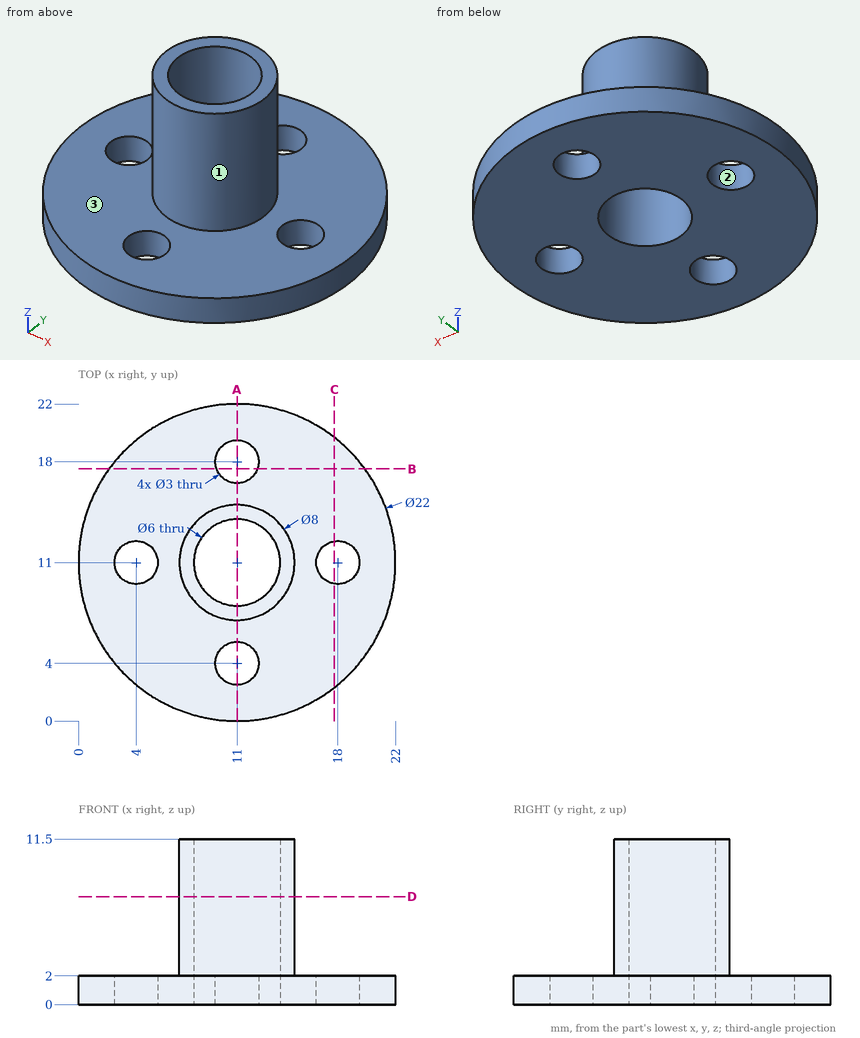
Input: dimensioned drawing with shaded views. Units: mm. Origin: part minimum x, y, z. Give positions to 0.01 mm unless a question says otherwise; leave off trailing zeros. Order: outer loops, then holes, each group sorted by start corner. A loop starts at its lowest first (then second) coordinate and runs counter-clockwise, first axis right, second up. Notation, with made-up numbers: (29, 72.25) -> (88, 72.25) arc R23 ccw to (88, 87.25) -> close; hole circle Ø7 at (-34, 40.25). An arc over 180 degrees is marked (long way). Use a Markdown table: item, result.
1) Section query B-B, the plane y = 17.5. Return the cut outline in (x, z), then the cut area to 3 significant figures.
Answer list:
| item | result |
|---|---|
| outline | (2.13, 0) -> (9.59, 0) -> (9.59, 2) -> (2.13, 2) -> close; (12.41, 0) -> (19.87, 0) -> (19.87, 2) -> (12.41, 2) -> close |
| area | 29.8 mm² |
2) Section query C-C, the plane x = 17.75. Return the cut outline in (y, z), then the cut area to 3 significant figures.
Answer list:
| item | result |
|---|---|
| outline | (2.31, 0) -> (9.52, 0) -> (9.52, 2) -> (2.31, 2) -> close; (12.48, 0) -> (19.69, 0) -> (19.69, 2) -> (12.48, 2) -> close |
| area | 28.8 mm² |
3) Mould query, pull axis Y, two halves, no side actions, for the marked faces 1, 2 and 3. Classes: +Y half, -Y half, draft (parallel to the pull), parting line (faces both ways), or undercut.
Answer list:
| item | result |
|---|---|
| face 1 | parting line |
| face 2 | undercut |
| face 3 | draft |
4) Section query D-D, the plane z = 7.5. Return the cut outline in (x, y), then the cut area to 3 significant figures.
Answer list:
| item | result |
|---|---|
| outline | circle Ø8 at (11, 11); hole circle Ø6 at (11, 11) |
| area | 22.0 mm² |
5) Contact query for flat-ended pins moving along their axis: P1, Ø1, axis at x = 19.5, z = 3, coming from the -Y side; P2, Ø3, axis at y = 18.5, z = 1.5, coming from the -X side; P3, Ø6, axis at x = 11, z = 5.5, coming from the -Y side; P4, Ø1, axis at y = 14, z = 2, coming from the +X side. Output: stop coordinate, or through.
Answer list:
| item | result |
|---|---|
| P1 | through |
| P2 | x = 1.78 |
| P3 | y = 7 |
| P4 | x = 21.71 |
6) Ray query, line 1 along Y through (x, z) = (11, 1.55); line 2 along Z through (x, y) = (14.25, 14); line 3 along X through (y, z) = (12.75, 1.25). Return the intervals inside material, ascending. Write a range as [from, to].
Answer list:
| item | result |
|---|---|
| line 1 | [0, 2.5], [5.5, 8], [14, 16.5], [19.5, 22] |
| line 2 | [0, 2] |
| line 3 | [0.14, 8.56], [13.44, 21.86] |
7) Section query A-A, the plane x = 11. Return the cut outline in (y, z).
Answer list:
| item | result |
|---|---|
| outline | (0, 0) -> (2.5, 0) -> (2.5, 2) -> (0, 2) -> close; (5.5, 0) -> (8, 0) -> (8, 11.5) -> (7, 11.5) -> (7, 2) -> (5.5, 2) -> close; (14, 0) -> (16.5, 0) -> (16.5, 2) -> (15, 2) -> (15, 11.5) -> (14, 11.5) -> close; (19.5, 0) -> (22, 0) -> (22, 2) -> (19.5, 2) -> close |
